Design review of the part built by this model. Coordinates are the model's own, in mm. A direction names the side the tool comes from. Give positions to 0.01 mm unless a question says otherwise; leave off trailing zeros. Write each loop counter-clockwise with the first axis right and the second up, starting at its lowest first coordinate (ties: lowest second). Pieces come first, ordered by that corner, then holes. Notation, with made-up numbers: (54.5, 4) - (107.5, 4) arc R25 ccw to (107.5, 28) - close; hole circle Ø4 at (-10.75, 46.5). An arc over 180 degrees is marked (long way). Use a Markdown table: item, result. Add a question column.
```python
from build123d import *

# Parameters (mm, degrees)
SKETCH1_W           = 52
SKETCH1_H           = 22
BOSS_EXTRUDE1_DEPTH = 3
SKETCH2_W           = 3
SKETCH2_H           = 3
BOSS_EXTRUDE2_DEPTH = 3
SKETCH3_W           = 3
SKETCH3_H           = 3
BOSS_EXTRUDE3_DEPTH = 3
SKETCH4_W           = 10.5
SKETCH4_H           = 3
BOSS_EXTRUDE4_DEPTH = 3
SKETCH5_W           = 35
SKETCH5_H           = 1.5
CUT_EXTRUDE1_DEPTH  = 3
SKETCH6_W           = 22.5
SKETCH6_H           = 2.539151914
CUT_EXTRUDE2_DEPTH  = 3


with BuildPart() as part:
    # Sketch1 → Boss-Extrude1 (new body)
    with BuildSketch(Plane.XY):
        Rectangle(SKETCH1_W, SKETCH1_H)
    extrude(amount=BOSS_EXTRUDE1_DEPTH)

    # Sketch2 → Boss-Extrude2 (add)
    with BuildSketch(Plane.ZY.offset(26)):
        with Locations((1.5, 6.5)):
            Rectangle(SKETCH2_W, SKETCH2_H)
        with Locations((1.5, -6.5)):
            Rectangle(SKETCH2_W, SKETCH2_H)
    extrude(amount=BOSS_EXTRUDE2_DEPTH)

    # Sketch3 → Boss-Extrude3 (add)
    with BuildSketch(Plane(origin=(26, 0, 0), x_dir=(0, 0, -1), z_dir=(1, 0, 0))):
        with Locations((-1.5, 6.5)):
            Rectangle(SKETCH3_W, SKETCH3_H)
        with Locations((-1.5, -6.5)):
            Rectangle(SKETCH3_W, SKETCH3_H)
    extrude(amount=BOSS_EXTRUDE3_DEPTH)

    # Sketch4 → Boss-Extrude4 (add)
    with BuildSketch(Plane.XZ.offset(11)):
        with Locations((-15.5, 1.5)):
            Rectangle(SKETCH4_W, SKETCH4_H)
        with Locations((15.5, 1.5)):
            Rectangle(SKETCH4_W, SKETCH4_H)
    extrude(amount=BOSS_EXTRUDE4_DEPTH)

    # Sketch5 → Cut-Extrude1 (cut)
    with BuildSketch(Plane.XY.offset(3)):
        with Locations((0, -5.25)):
            Rectangle(SKETCH5_W, SKETCH5_H)
    extrude(amount=-CUT_EXTRUDE1_DEPTH, mode=Mode.SUBTRACT)

    # Sketch6 → Cut-Extrude2 (cut)
    with BuildSketch(Plane.XY.offset(3)):
        with Locations((4.75, -7.269575957)):
            Rectangle(SKETCH6_W, SKETCH6_H)
    extrude(amount=-CUT_EXTRUDE2_DEPTH, mode=Mode.SUBTRACT)


solid = part.part
```
(1) Add section B-B (x = -8). State the section outline as (y, z) points, and give its area (3 significant figures).
(2) For line 1 along Y through (x, z) = (2.5, 0.4); line 2 along X through (y, z) = (-11.25, 0.9); line 3 along X through (y, z) = (-6.25, 2.7), list the stretches that pass through material, from the lowest coordinate up.
(3) Add section D-D (x = 23). State the section outline as (y, z) points, and give its area (3 significant figures).
(4) Add section A-A (y = -12.5). State the section outline as (x, z) points, and give its area (3 significant figures).
(5) Add section C-C (y = -2.5). State the section outline as (x, z) points, and give its area (3 significant figures).
(6) Mouldability with a two-part tool opening along X and no side actions: class faces 5 (the face through (0, -1, 3)), 6 (the face through (29, -6, 2)), 7 (the face through (10.25, -12, 1)) as +X half, -X half, draft (parallel to the pull), parting line (faces both ways), or undercut.
(7) Insertion check: pin 1 (1.5 mm diameter, centred on y = -12, z = 2, fed in from +X); pin 2 (1.5 mm diameter, centred on y = -2.5, z = 1, fed in from -X); pin 3 (0.9 mm diameter, centred on x = 23.5, z = 1.5, fed in from -Y). Each pin has a flat end and moves straight along its axis. Give the tip position at first contact, or say it passes through.
(8) Tool access review of faces 1 (the face through (27, -8, 2)), 2 (the face through (27, 5, 2)), 3 (the face through (-23, -11, 1)), 4 (the face through (17, -6, 2)): name each direction out of +Z, -Z, +X, -X, +Y, -Y from which nothing blocks a thin tool from reaching the whole face with its end or side.
Answers follow:
| question | item | result |
|---|---|---|
| 1 | outline | (-11, 0) - (-6, 0) - (-6, 3) - (-11, 3) - close; (-4.5, 0) - (11, 0) - (11, 3) - (-4.5, 3) - close |
| 1 | area | 61.5 mm^2 |
| 2 | line 1 | -11 to -8.54, -4.5 to 11 |
| 2 | line 2 | -20.75 to -10.25, 10.25 to 20.75 |
| 2 | line 3 | -29 to -6.5, 16 to 29 |
| 3 | outline | (-11, 0) - (11, 0) - (11, 3) - (-11, 3) - close |
| 3 | area | 66.0 mm^2 |
| 4 | outline | (-20.75, 0) - (-10.25, 0) - (-10.25, 3) - (-20.75, 3) - close; (10.25, 0) - (20.75, 0) - (20.75, 3) - (10.25, 3) - close |
| 4 | area | 63.0 mm^2 |
| 5 | outline | (-26, 0) - (26, 0) - (26, 3) - (-26, 3) - close |
| 5 | area | 156 mm^2 |
| 6 | face 5 | draft |
| 6 | face 6 | +X half |
| 6 | face 7 | undercut |
| 7 | pin 1 | x = 20.75 |
| 7 | pin 2 | x = -26 |
| 7 | pin 3 | y = -11 |
| 8 | face 1 | +Z, -Z, +X, -Y |
| 8 | face 2 | +Z, -Z, +X |
| 8 | face 3 | +Z, -Z, -X, -Y |
| 8 | face 4 | +Z, -Z |
